Study the drawing (mm; zero at the part's minimum x, y, z) and answer. A direction names the side the tool comes from. Coordinates: 2 decimals unless noted, no trailing zeros. Loops run counter-clockwise (first coordinate to the right, second up) from the corner with the lowest first, then second, coordinate; pieces in that order, holes last. Notation, with made-up numbers: M 51.5,35.5 L 76.5,35.5 A11 ccw 76.5,39.5 Z; hole C -14,-25 d3. An arc over 180 degrees is marked long. Use one line per item in the form item = value. Start each with the question number.
1. Flat-ended cylindrical pins translate along their axes: pin 1 (1.5 mm diameter, centred on y = 38, z = 4, fed in from -X); pin 2 (9 mm diameter, centred on x = 60, y = 52, fed in from +Z); pin 3 (22.5 mm diameter, centred on x = 48.5, y = 52.5, fed in from +Z). Find the tip coordinate at first contact, or state that the pin passes through.
2. The part is cut by section D-D (x = 45). Give the vertices of the cut face in (y, z), plus the area to 3 significant figures.
3. The part is cut by section A-A (x = 61.5). Give the vertices of the cut face in (y, z), plus the area to 3 significant figures.
4. The part is cut by section B-B (z = 8). Give the vertices of the cut face in (x, y).
5. For a pull along X with two mould halves and no side action, classify the marked faces 3, 4 and 5 as released by +X, released by -X, zero draft, split by the parting line, or undercut.
6. Find the intervals of material crossed by probe 1 along X at (y, z) = (72.5, 1.25); probe 2 along X at (y, z) = (57, 2.5); probe 3 along Y at (x, z) = (19.5, 4), in increasing order. Write a range as [from, to].
7. A tool of negligible diameter and unlimited length cuts with its end or side. For the marked faces 1 and 2, from which of +Z, -Z, +X, -X, +Y, -Y can it reach the whole face along a straight path? Write none if from no direction.
8. The part is cut by section C-C (y = 13). Give the vertices of the cut face in (x, z).
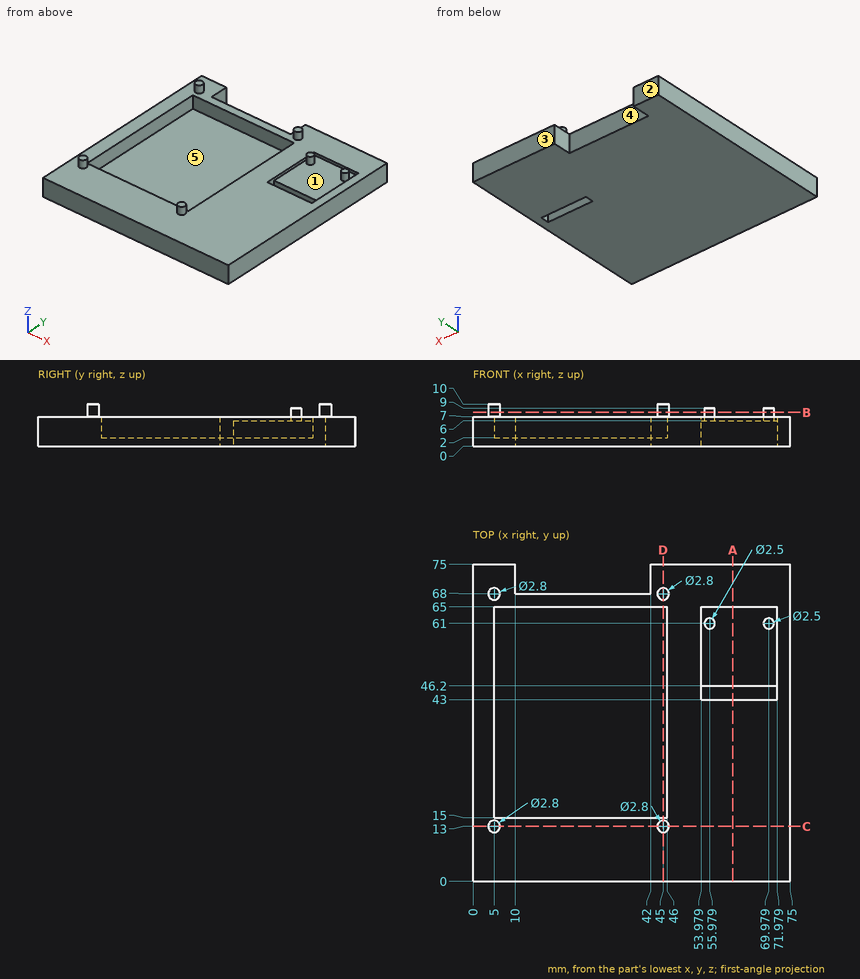
Computed values:
q1.pin_1 = 0
q1.pin_2 = 6
q1.pin_3 = 9
q2.outline = M 0,0 L 75,0 L 75,7 L 69.4,7 L 69.4,10 L 66.6,10 L 66.6,7 L 65,7 L 65,2 L 15,2 L 15,7 L 14.4,7 L 14.4,10 L 11.6,10 L 11.6,7 L 0,7 Z
q2.area = 292 mm²
q3.outline = M 0,0 L 43,0 L 43,7 L 0,7 Z; M 46.2,0 L 75,0 L 75,7 L 65,7 L 65,6 L 46.2,6 Z
q3.area = 484 mm²
q4.outline = C 5,13 d2.8; C 5,68 d2.8; C 45,13 d2.8; C 45,68 d2.8; C 55.98,61 d2.5; C 69.98,61 d2.5
q5.face_3 = zero draft
q5.face_4 = undercut
q5.face_5 = undercut
q6.probe_1 = [0, 10], [42, 75]
q6.probe_2 = [0, 5], [46, 75]
q6.probe_3 = [0, 15], [65, 68]
q7.face_1 = +Z
q7.face_2 = +Z, -Z, +X, -X, +Y
q8.outline = M 0,0 L 75,0 L 75,7 L 46.4,7 L 46.4,10 L 43.6,10 L 43.6,7 L 6.4,7 L 6.4,10 L 3.6,10 L 3.6,7 L 0,7 Z
